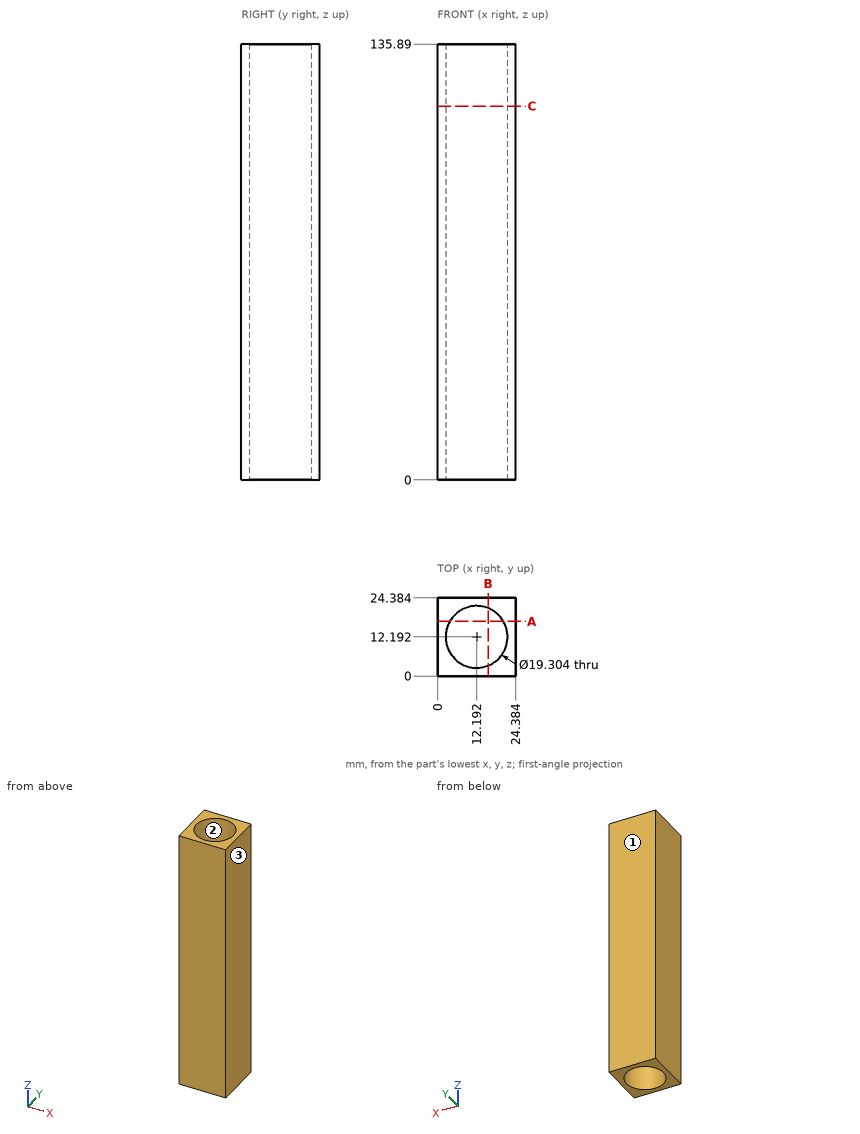
Drawing for the job (mm, zero at the part's lowest x, y, z). Coordinates: 2 decimals unless noted, no trailing zeros. Write each loop counter-clockwise with the first axis right and the second up, starting at its lowest first coordinate (ties: lowest second). Pieces come first, ordered by that corner, then holes. Notation, with made-up numbers: (-3.75, 49.25) -> (35.25, 49.25) arc R23 cw to (35.25, 69.25) -> close; hole circle Ø11 at (-19, 69.5). An arc over 180 degrees is marked (long way). One line per item, written item: value. Start each with the question number.
1) Flat gauge pin, fed straight in: pin 1 Ø2 at (x, z) = (16, 85.5) entering from -Y. Where does the tip first touch, or does it go through?
2) Slice it at C-C on z = 116.5. Write the cut outline in (x, y), then the cut area to 3 significant figures.
3) Pull direction Y, two halves, no side cores. Call the marked faces 1, 2 and 3: +Y half, -Y half, draft (parallel to the pull), parting line (faces both ways), or undercut.
4) Slice it at B-B on x = 15.75. Write the cut outline in (y, z), then the cut area to 3 significant figures.
5) Slice it at A-A on y = 17. Write the cut outline in (x, z), then the cut area to 3 significant figures.
6) Probe probe 1 along Y at (x, z) = (12.75, 41); probe 2 along Y at (x, z) = (12.25, 68); probe 3 along X at (y, z) = (17, 37.5). List the from-to ranges inside material, lowest first.
Answers follow:
1. pin 1: y = 0
2. outline: (0, 0) -> (24.38, 0) -> (24.38, 24.38) -> (0, 24.38) -> close; hole circle Ø19.3 at (12.19, 12.19)
2. area: 302 mm2
3. face 1: +Y half
3. face 2: undercut
3. face 3: draft
4. outline: (0, 0) -> (3.22, 0) -> (3.22, 135.89) -> (0, 135.89) -> close; (21.16, 0) -> (24.38, 0) -> (24.38, 135.89) -> (21.16, 135.89) -> close
4. area: 875 mm2
5. outline: (0, 0) -> (3.82, 0) -> (3.82, 135.89) -> (0, 135.89) -> close; (20.56, 0) -> (24.38, 0) -> (24.38, 135.89) -> (20.56, 135.89) -> close
5. area: 1,040 mm2
6. probe 1: 0 to 2.56, 21.83 to 24.38
6. probe 2: 0 to 2.54, 21.84 to 24.38
6. probe 3: 0 to 3.82, 20.56 to 24.38
